```python
from build123d import *

# Parameters (mm, degrees)
F0_W     = 5
F0_H     = 2.5
F1_DEPTH = 2.8
F3_DEPTH = 38
F5_DEPTH = 40


with BuildPart() as f1:
    # F0 (on Front) → F1 (new body)
    with BuildSketch(Plane.XZ):
        with Locations((-13.717596, 1.25)):
            Rectangle(F0_W, F0_H)
        with Locations((13.717596, 1.25)):
            Rectangle(F0_W, F0_H)
        with Locations((-13.717596, -40.75)):
            Rectangle(F0_W, F0_H)
        with Locations((13.717596, -40.75)):
            Rectangle(F0_W, F0_H)
        Polygon((11.217596, 0), (0, 0), (-11.217596, 0), (-16.217596, 0), (-19, 0), (-19, -39.5), (-16.217596, -39.5), (-11.217596, -39.5), (0, -39.5), (11.217596, -39.5), (16.217596, -39.5), (19, -39.5), (19, 0), (16.217596, 0), align=None)
    extrude(amount=F1_DEPTH)

    # F2 (on face) → F3 (join)
    with BuildSketch(Plane(origin=(-19, 0, 0), x_dir=(0, -1, 0), z_dir=(-1, 0, 0))):
        Polygon((2.8, 0), (2.8, -39.5), (32.8, -39.5), (22.8, 0), align=None)
    extrude(amount=-F3_DEPTH)

    # F4 (on face) → F5 (cut)
    with BuildSketch(Plane.XZ):
        Polygon((-5, -29.5), (-5, -39.5), (0, -39.5), (5, -39.5), (5, -29.5), align=None)
    extrude(amount=F5_DEPTH, mode=Mode.SUBTRACT)


solid = f1.part
```
Source: CAD feature listing. Evaluate the final solid. Frame: model axes, mm. A direction names the side the tool comes from. Give positions to 0.01 mm unless a question says otherwise; leave off trailing zeros. Write each loop counter-clockwise with the first axis right and the second up, starting at its lowest first coordinate (ties: lowest second). Pieces come first, ordered by that corner, then holes. Notation, with made-up numbers: (88.5, 57) - (146.5, 57) arc R21 ccw to (146.5, 62) - close; hole circle Ø8 at (63.25, 34). An arc over 180 degrees is marked (long way). One line per item, written item: value. Start each with the question number.
Q1. First-contact query: pin 1 Ø10 at (x, z) = (-4.5, -19.5) entering from -Y; pin 2 Ø5 at (x, y) = (-2, -11) entering from -Z; pin 3 Ø5 at (x, z) = (14.5, -12.5) entering from -Y; pin 4 Ø4 at (x, z) = (-2.5, -36) entering from +Y. Flat tips, straight axial feed; report the tip coordinate or a pass-through.
Q2. Section query B-B, the plane y = -5.5. Return the cut outline in (x, z), then the cut area to 3 significant figures.
Q3. Material intervals for probe 1 along X at (y, z) = (-1, -31); probe 2 along Z at (x, y) = (0, -6); probe 3 along Z at (x, y) = (5.5, -16.5), sorted ascending. Write a range as from..to.
Q4. Section query C-C, the plane x = 12. Return the cut outline in (y, z), then the cut area to 3 significant figures.
Q5. Set-up query: faces 5 (the face through (-16.218, -1, 1)), 6 (the face through (-11.218, -1, 1)), 7 (the face through (16.218, -1, -41)), 8 (the face through (11.218, -1, -41)). Return all of +Z, -Z, +X, -X, +Y, -Y with unobstructed straight access to the full face (end or side cutting, diameter ignored); none if empty.
Q6. Draft query along X for faces 1 (the face through (-5, -16, -34)), 2 (the face through (16.218, -1, 1)), 3 (the face through (14, -2.8, -41)), 4 (the face through (11.218, -1, 1)). Return one class per face: +X half, -X half, draft (parallel to the pull), parting line (faces both ways), or undercut.
Q7. Section query D-D, the plane z = -14. Return the cut outline in (x, y), then the cut area to 3 significant figures.
Q8. Section query A-A, the plane z = -36. Return the cut outline in (x, y), then the cut area to 3 significant figures.
Answer:
1. pin 1: stops at y = -29
1. pin 2: stops at z = -29.5
1. pin 3: stops at y = -26.6
1. pin 4: passes through
2. outline: (-19, -39.5) - (-5, -39.5) - (-5, -29.5) - (5, -29.5) - (5, -39.5) - (19, -39.5) - (19, 0) - (-19, 0) - close
2. area: 1,400 mm2
3. probe 1: x = -19..-5, 5..19
3. probe 2: z = -29.5..0
3. probe 3: z = -39.5..0
4. outline: (-32.8, -39.5) - (-2.8, -39.5) - (-2.8, -42) - (0, -42) - (0, 2.5) - (-2.8, 2.5) - (-2.8, 0) - (-22.8, 0) - close
4. area: 1,110 mm2
5. face 5: +Z, -X, +Y, -Y
5. face 6: +Z, +Y, -Y
5. face 7: -Z, +X, +Y, -Y
5. face 8: -Z, +Y, -Y
6. face 1: undercut
6. face 2: +X half
6. face 3: draft
6. face 4: undercut
7. outline: (-19, -26.34) - (19, -26.34) - (19, 0) - (-19, 0) - close
7. area: 1,000 mm2
8. outline: (-19, -31.91) - (-5, -31.91) - (-5, 0) - (-19, 0) - close; (5, -31.91) - (19, -31.91) - (19, 0) - (5, 0) - close
8. area: 894 mm2
